Geometry: final body of the model. Coordinates: model frame, mm. A direction names the side the tool comes from. Give positions to 0.01 mm unless a question says otherwise; leave off trailing zeros. Write each loop counter-clockwise with the first axis right and the second up, starting at its lowest first coordinate (ties: lowest second). Pieces come first, ordered by that corner, then holes. Notation, with made-up numbers: (46, 39.25) -> (105, 39.25) arc R22 ccw to (105, 63.25) -> close; hole circle Ø1 at (-4, 52.5). An arc over 180 degrees is marked (long way). Answer as a JSON object with one key per item and string values. Group by question number.
(1) Section query B-B on z = 0. Output: boundary loops of the cut face in (x, y) (3 decimals).
(2) Contact query for flat-ended pins moving along their axis: pin 1 Ø1.5 at (x, y) = (14.5, -1) entering from +Z; pin 2 Ø2 at (x, y) = (8, -2.5) entering from +Z; pin 3 Ø4 at (x, z) = (18, 2) entering from +Y. Output: stop coordinate, or through.
(3) Section query D-D on y = 1.5. Output: boundary loops of the cut face in (x, z) (1 decimal).
(4) Section query C-C on x = 9.5. Output: boundary loops of the cut face in (y, z) (3 decimals).
(5) Section query A-A on y = 0. Output: boundary loops of the cut face in (x, z) (3 decimals), plus the area to 3 significant figures.
(6) Material intervals for probe 1 along X at (y, z) = (4, -1.5); probe 2 along X at (y, z) = (2.5, 3.75); probe 3 along Z at (x, y) = (11, 0) (3 decimals), sorted ascending.
(7) Set-up query: faces 1 (the face through (25.019, 0, 0)), 2 (the face through (8.93, 3.1, -0.69)), 3 (the face through (1.27, 0, 4)), 4 (the face through (1.27, 0, -4)). Return all of +Z, -Z, +X, -X, +Y, -Y with unobstructed straight access to the full face (end or side cutting, diameter ignored); none if empty.
from build123d import *

# Parameters (mm, degrees)
F4_DEPTH = 3.81


with BuildPart() as f1:
    # F0 (on Front) → F1 (revolve)
    with BuildSketch(Plane.XZ):
        Polygon((0, 5.08), (0, 0), (25.019, 0), (25.019, 2.413), (15.494, 2.413), (15.494, 3.175), (2.54, 3.175), (2.54, 5.08), align=None)
    revolve(axis=Axis((12.5095, 0, 0), (1, 0, 0)))

    # F3 (on offset) → F4 (cut)
    with BuildSketch(Plane.YZ.offset(-2.54)):
        Polygon((-5.874861, 3.175), (0, 3.175), (5.874861, 3.175), (5.874861, 6.309091), (-5.874861, 6.309091), align=None)
        Polygon((5.874861, -3.175), (0, -3.175), (-5.874861, -3.175), (-5.874861, -6.309091), (5.874861, -6.309091), align=None)
    extrude(amount=F4_DEPTH, mode=Mode.SUBTRACT)


solid = f1.part
Answer list:
{
 "1": {"outline": "(0, -5.08) -> (2.54, -5.08) -> (2.54, -3.175) -> (15.494, -3.175) -> (15.494, -2.413) -> (25.019, -2.413) -> (25.019, 2.413) -> (15.494, 2.413) -> (15.494, 3.175) -> (2.54, 3.175) -> (2.54, 5.08) -> (0, 5.08) -> close"},
 "2": {"pin 1": "z = 3.17", "pin 2": "z = 2.8", "pin 3": "y = 2.41"},
 "3": {"outline": "(0, -3.2) -> (1.3, -3.2) -> (1.3, -4.9) -> (2.5, -4.9) -> (2.5, -2.8) -> (15.5, -2.8) -> (15.5, -1.9) -> (25, -1.9) -> (25, 1.9) -> (15.5, 1.9) -> (15.5, 2.8) -> (2.5, 2.8) -> (2.5, 4.9) -> (1.3, 4.9) -> (1.3, 3.2) -> (0, 3.2) -> close"},
 "4": {"outline": "circle Ø6.35 at (0, 0)"},
 "5": {"outline": "(0, -3.175) -> (1.27, -3.175) -> (1.27, -5.08) -> (2.54, -5.08) -> (2.54, -3.175) -> (15.494, -3.175) -> (15.494, -2.413) -> (25.019, -2.413) -> (25.019, 2.413) -> (15.494, 2.413) -> (15.494, 3.175) -> (2.54, 3.175) -> (2.54, 5.08) -> (1.27, 5.08) -> (1.27, 3.175) -> (0, 3.175) -> close", "area": "149 mm2"},
 "6": {"probe 1": "0 to 2.54", "probe 2": "1.27 to 2.54", "probe 3": "-3.175 to 3.175"},
 "7": {"face 1": "+Z, -Z, +X, +Y, -Y", "face 2": "+X", "face 3": "+Z, -X, +Y, -Y", "face 4": "-Z, -X, +Y, -Y"}
}
